Autodesk Inventor part; units mm, degrees
ref_plane "YZ Plane" through (0, 0, 0) normal (1, 0, 0) x (0, 1, 0)
ref_plane "XY Plane" through (0, 0, 0) normal (0, 0, 1) x (1, 0, 0)
sketch "Block1" plane through (0, 0, 0) normal (0, 0, 1) x (1, 0, 0)
  line L0 (-13, 33) -> (0, 33)
  line L1 (0, 33) -> (0, 31.984)
  line L2 (0, 0) -> (-7.5, 0)
  line L3 (-5.5, 31.984) -> (0, 31.984)
  spline S0 degree 4 poles (-5.5, 31.984) (-8.3018, 31.984) (-14.9701, 28.615) (-2.778, 19.5085) (-12.1324, 9.4997) (-13.0429, 3.8555) (-13.0429, 0) knots 0 0 0 0 0 0.349618 0.599618 1 1 1 1 1
  spline S1 degree 4 poles (-5.5, 33) (-8.695, 33) (-16.2444, 29.0645) (-3.8371, 19.8287) (-13.0244, 9.853) (-14.2875, 3.9571) (-14.2875, 0) knots 0 0 0 0 0 0.356198 0.606198 1 1 1 1 1
  line L4 (-13.0429, 0) -> (13.0429, 0)
  line L5 (13.0429, 0) -> (13.0429, -90)
  line L6 (13.0429, -90) -> (-13.0429, -90)
  line L7 (-13.0429, -90) -> (-13.0429, 0)
  line L8 (0, 33) -> (0, 31.984)
  line L9 (0, 0) -> (14.2875, 0)
  line L10 (14.2875, 0) -> (14.2875, -90)
  line L11 (14.2875, -90) -> (-14.2875, -90)
  line L12 (-14.2875, -90) -> (-14.2875, 0)
  line L13 (-14.2875, 0) -> (-13.0429, 0)
  line L14 (-13.0429, 0) -> (-12.0269, 0)
  line L15 (-12.0269, 0) -> (-12.0269, -5)
  line L16 (-12.0269, -5) -> (-13.0429, -5)
  line L17 (-13.0429, -5) -> (-13.0429, 0)
  spline S2 degree 4 poles (-12.0269, 0) (-12.0269, 1.8651) (-12.9196, 3.9842) (-12.4898, 5.3301) (-12.0051, 6.8202) knots 0 0 0 0 0 1 1 1 1 1
  point P0 (-5.8286, -1.9888)
  point P1 (-2.75, 31.984)
  point P2 (-10.8475, 28.6822)
  point P3 (-8.5755, 20.4298)
  point P4 (-10.7949, 9.9764)
  point P5 (-11.8109, 29.0047)
  point P6 (-9.5915, 20.5086)
  point P7 (-11.8109, 10.2944)
  point P8 (-12.757, 3.7934)
  point P9 (-12.2202, 6.1237)
  point P10 (-12.4905, 4.0174)
  dimension "d0" = 1.016
  dimension "d1" = 1.016
  dimension "d2" = 1.016
  dimension "d3" = 1.016
  dimension "d4" = 90
  dimension "d5" = 26.0858
  dimension "d6" = 33
  dimension "d7" = 5.5
  dimension "d8" = 28.575
  dimension "d9" = 5
  dimension "d10" = 1.016
sketch "Sketch2" plane through (0, 0, 0) normal (1, 0, 0) x (0, 1, 0)
  point P0 (0, 0)
sketch "Sketch3" plane through (0, 0, 0) normal (1, 0, 0) x (0, 1, 0)
  line L0 (0, -114.856) -> (0, 59.1357)
  line L1 (0, 29) -> (-11.8121, 29)
  line L2 (-13.0429, 0) -> (-12.0429, 0)
  line L3 (-12.0429, 0) -> (-12.0429, -3)
  line L4 (-12.0429, -3) -> (-13.0429, -3)
  line L5 (-13.0429, -3) -> (-13.0429, 0)
  line L6 (-14.2875, 0) -> (-14.2875, -7.5209)
  spline S0 degree 4 poles (-8.7178, 15.3035) (-9.5873, 11.2411) (-11.424, 6.9381) (-12.0429, 3.6863) (-12.0429, 0) knots 0 0 0 0 0 1 1 1 1 1
  spline S1 degree 4 poles (-11.8121, 29) (-11.4923, 26.2408) (-6.533, 15.3028) (-13.5295, 15.4591) (-14.2875, 3.7094) (-14.2875, 0) knots 0 0 0 0 0 0.596386 1 1 1 1 1
  line L7 (-14.2875, 0) -> (-13.0429, 0)
  line L8 (0, 29) -> (-11.625, 29)
  line L9 (-11.625, 28) -> (0, 28)
  line L10 (0, 28) -> (0, 29)
  line L11 (-6, 28) -> (-8.7178, 15.3035)
  point P0 (0, 0)
  point P1 (-12.0269, 0)
  point P2 (-6, 29)
  point P3 (-11.1126, 6.8247)
  point P4 (-10.2731, 22.7051)
  point P5 (-10.2729, 16.6704)
  point P6 (-12.5423, 11.3252)
  dimension "d12" = 29
  dimension "d13" = 14.2875
  dimension "d14" = 3
  dimension "d15" = 1
  dimension "d17" = 13.0429
  dimension "d18" = 1
  dimension "d35" = 6
revolve "Revolution1" add sketch "Sketch3" angle 360 about axis through (0, 0, -10) along (0, 0, 1)
fillet "Fillet1" radius 2 1 edges at (0, 11.8121, 29)
fillet "Fillet2" [suppressed]
hole "Hole1" at (0, 0, 29) direction (0, 0, -1) diameter 12 end through all
ref_plane "Work Plane2" through (0, 8.3, 0) normal (0, 1, 0) x (-1, 0, 0)
sketch "Sketch6" plane through (0, 8.3, 0) normal (0, 1, 0) x (-1, 0, 0)
  arc A0 (2.6663, 15.3035) -> (-2.6663, 15.3035) centre (-2.6663, 15.3035) ccw
  arc A1 (-2.6663, 15.3035) -> (-8.7259, 0) centre (-8.7259, 0) ccw
  line L0 (-8.7259, 0) -> (-8.7259, -3)
  line L1 (-8.7259, -3) -> (-10.0612, -3)
  line L2 (-10.0612, -3) -> (-10.0612, 0)
  line L3 (-10.0612, 0) -> (-11.6294, 0)
  arc A2 (-11.6294, 0) -> (-7.5554, 26.4676) centre (-7.5554, 26.4676) ccw
  arc A3 (-7.5554, 26.4676) -> (-4.1863, 29) centre (-4.1863, 29) ccw
  line L4 (-4.1863, 29) -> (4.1863, 29)
  arc A4 (4.1863, 29) -> (7.5554, 26.4676) centre (7.5554, 26.4676) ccw
  arc A5 (7.5554, 26.4676) -> (11.6294, 0) centre (11.6294, 0) ccw
  line L5 (11.6294, 0) -> (10.0612, 0)
  line L6 (10.0612, 0) -> (10.0612, -3)
  line L7 (10.0612, -3) -> (8.7259, -3)
  line L8 (8.7259, -3) -> (8.7259, 0)
  arc A6 (8.7259, 0) -> (2.6663, 15.3035) centre (2.6663, 15.3035) ccw
  line L9 (12.0429, -3) -> (-12.0429, -3)
  line L10 (0, -114.856) -> (0, 59.1357)
  line L11 (-10, 8) -> (10, 8)
  line L12 (10, 8) -> (10, -3)
  line L13 (10, -3) -> (-10, -3)
  line L14 (-10, -3) -> (-10, 8)
  point P0 (0, 0)
  point P1 (0, 8)
  dimension "d46" = 11
  dimension "d47" = 20
extrude "Extrusion1" cut sketch "Sketch6" along normal through all contours L11 L12 A2 L10 | L10 A2 L0 A1 L14 L11 | L10 L9 L0 A2 | A2 L12 A6 L8 L9 L10 | A2 A1 L0 | L0 L1 L14 A1 A2 | A2 A1 L14 | L8 A6 L12 L7
equation "\"d0\" = d11"
equation "\"d11\" = 1.016"
properties part number "New" material "Stainless Steel"
Model file for the job. Use its own axes, mm. A direction names the side the tool comes from. Coordinates: 2 decimals unless noted, no trailing zeros. Write each question's results on one line, items separated by ' | '. Start each with the question number.
1) Probe line 1 along X through (y, z) = (0, 28.4); line 2 along X through (y, z) = (0, 28.7); line 3 along Y through (x, z) = (0, 28.3). List the from-to ranges inside material, lowest first. Write a range as from..to.
2) Mould opens along X. For faces 1 (the face through (-9, 8.3, 4)), 2 (the face through (3, -12, -3)) say: pulls with the +X half, pulls with the -X half, needs draft (parallel to the pull), parting line crosses it, or undercut.
3) Flat gauge pins, fed straight in: P1, Ø3.5, axis at x = 8, z = 3.5, coming from the +Y side; P2, Ø1.6, axis at x = 4, y = 10, coming from the -Z side; P3, Ø2, axis at y = 9, z = 1.5, coming from the +X side. Where does each tip first touch, or does it go through?
4) 3-axis set-ups, long thin cutter, end or side, ignore diameter. For faces 3 (the face through (10, 9, 4)), 4 (the face through (-0.264, 5.994, 28.493)), 5 (the face through (-3, -13, 0)): which of +Z, -Z, +X, -X, +Y, -Y reach the whole face in a straight line?
Returned:
1) line 1: -10.72..-6, 6..10.72 | line 2: -10.35..-6, 6..10.35 | line 3: -10.82..-6, 6..10.82
2) face 1: undercut | face 2: needs draft
3) P1: y = 8.3 | P2: z = 8 | P3: x = 11.81
4) face 3: -Z, +Y | face 4: +Z, -Z | face 5: -Z
